Print and shaded views of the part. All mm, measured from the part's lowest x, y and z. Round coordinates to 2 decimals unless told otherwise and drop trailing zeros. Order: outer loops, then holes, each group sorted by start corner. A loop starts at its lowest first (then second) coordinate and runs counter-clockwise, first axis right, second up. Notation, with made-up numbers: (32, 51) -> (73, 51) arc R34 ccw to (73, 81) -> close; hole circle Ø10 at (23, -18.75). An arc over 180 degrees is marked (long way). Answer as CSV lines item,"result". Start each with the question number.
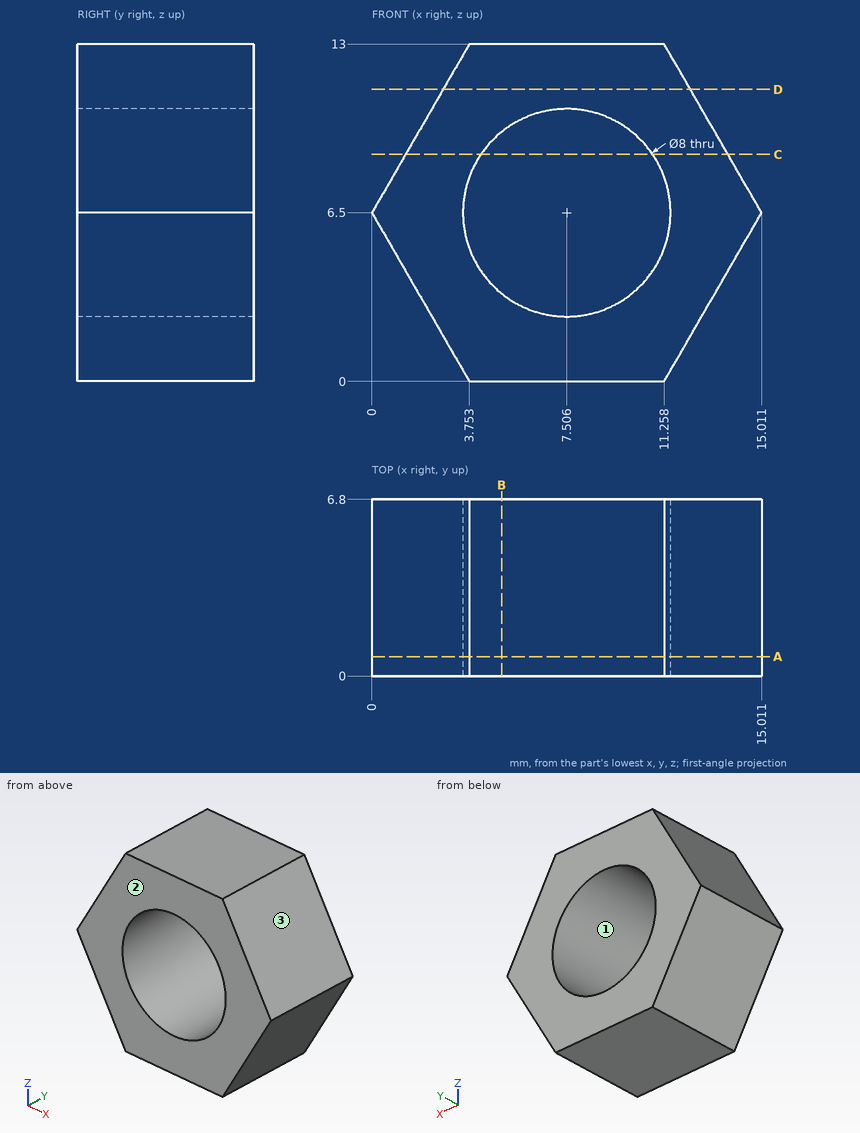
Item 1: Pin check, flat tips, straight feed: pin 1 (1.5 mm diameter, centred on y = 1.5, z = 4.5, fed in from -X); pin 2 (2 mm diameter, centred on y = 3, z = 4, fed in from +X) (1 decimal); pin 3 (4 mm diameter, centred on y = 5.5, z = 3.5, fed in from -X). Stop position of each tip, or through.
Item 2: Mould opens along X. For the marked faces 1, 2 and 3 say: released by +X, released by -X, zero draft, split by the parting line, or undercut.
Item 3: Band-saw the part on D-D, the plane z = 11.25. Give the cut face in (x, y).
Item 4: Band-saw the part on B-B, the plane x = 5. Give the cut face in (y, z), and give its area (3 significant figures).
Item 5: Band-saw the part on A-A, the plane y = 0.75. Give the cut face in (x, z) (1 decimal).
Item 6: Probe line 1 (X direction, y = 5.5, z = 7) (1 decimal); line 2 (Z direction, x = 8.5, y = 2.5) (1 decimal); line 3 (X direction, y = 4.25, z = 8.25). List the from-to ranges inside material, lowest first.
Item 7: Band-saw the part on C-C, the plane z = 8.75. Give the cut face in (x, y).
Values:
1,pin 1,"x = 0.72"
1,pin 2,"x = 14.1"
1,pin 3,"x = 0.58"
2,face 1,"undercut"
2,face 2,"zero draft"
2,face 3,"released by +X"
3,outline,"(2.74, 0) -> (12.27, 0) -> (12.27, 6.8) -> (2.74, 6.8) -> close"
4,outline,"(0, 0) -> (6.8, 0) -> (6.8, 3.38) -> (0, 3.38) -> close; (0, 9.62) -> (6.8, 9.62) -> (6.8, 13) -> (0, 13) -> close"
4,area,"46.0 mm²"
5,outline,"(0, 6.5) -> (3.8, 0) -> (11.3, 0) -> (15, 6.5) -> (11.3, 13) -> (3.8, 13) -> close; hole circle Ø8 at (7.5, 6.5)"
6,line 1,"0.3 to 3.5, 11.5 to 14.7"
6,line 2,"0 to 2.6, 10.4 to 13"
6,line 3,"1.01 to 3.91, 11.1 to 14"
7,outline,"(1.3, 0) -> (4.2, 0) -> (4.2, 6.8) -> (1.3, 6.8) -> close; (10.81, 0) -> (13.71, 0) -> (13.71, 6.8) -> (10.81, 6.8) -> close"
